Part print with two shaded views. Sizes in mm from the minimum x, y, z corner. Give positions to 0.01 mm unless a question says otherwise; leave off trailing zeros. Loops run counter-clockwise (first coordinate to the right, second up) from the corner with the lowest first, then second, coordinate; pieces in that order, holes last. Notation, with made-up numbers: M -16.5,21.5 L 19.5,21.5 A11 ccw 19.5,39.5 Z; hole C 37,-36.5 d7. An arc over 180 degrees is marked long. Answer in a Markdown table with one row per item.
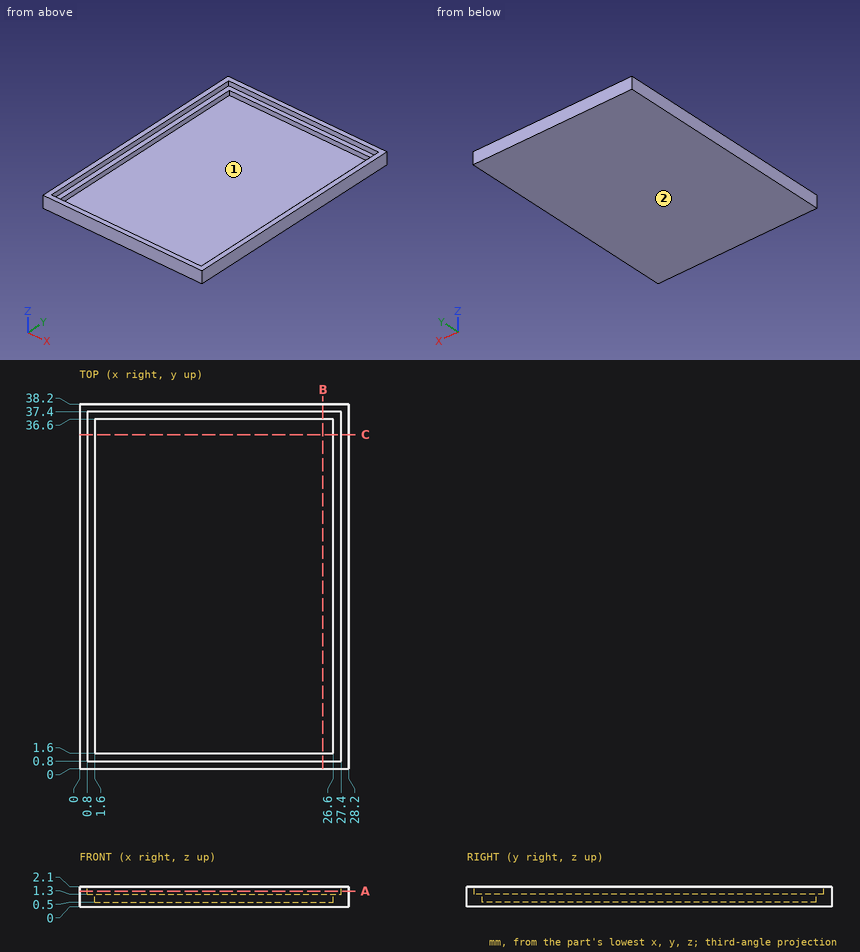
Q1. Saw through at A-A (z = 1.65). Give the cut face in (x, y), and give its area (3 significant figures).
Reported:
| item | result |
|---|---|
| outline | M 0,0 L 28.2,0 L 28.2,38.2 L 0,38.2 Z; hole M 0.8,0.8 L 27.4,0.8 L 27.4,37.4 L 0.8,37.4 Z |
| area | 104 mm² |
Q2. Saw through at B-B (x = 25.5). Give the cut face in (y, z).
Reported:
| item | result |
|---|---|
| outline | M 0,0 L 38.2,0 L 38.2,2.1 L 37.4,2.1 L 37.4,1.3 L 36.6,1.3 L 36.6,0.5 L 1.6,0.5 L 1.6,1.3 L 0.8,1.3 L 0.8,2.1 L 0,2.1 Z |
Q3. Drop flat-ended pins along their axis: pin 1 (1 mm diameter, centred on x = 12.5, z = 0.5, fed in from -Y); pin 2 (3 mm diameter, centred on x = 14.5, y = 24.5, fed in from +Z). Give the stop position or say it passes through.
Reported:
| item | result |
|---|---|
| pin 1 | y = 0 |
| pin 2 | z = 0.5 |
Q4. Probe probe 1 along X at (y, z) = (17.5, 1.4); probe 2 along Y at (x, z) = (23.75, 0.8); probe 3 along Y at (x, z) = (12.25, 1.5). List the from-to ranges inside material, lowest first.
Reported:
| item | result |
|---|---|
| probe 1 | 0 to 0.8, 27.4 to 28.2 |
| probe 2 | 0 to 1.6, 36.6 to 38.2 |
| probe 3 | 0 to 0.8, 37.4 to 38.2 |
Q5. Saw through at C-C (y = 35). Give the cut face in (x, z).
Reported:
| item | result |
|---|---|
| outline | M 0,0 L 28.2,0 L 28.2,2.1 L 27.4,2.1 L 27.4,1.3 L 26.6,1.3 L 26.6,0.5 L 1.6,0.5 L 1.6,1.3 L 0.8,1.3 L 0.8,2.1 L 0,2.1 Z |
Q6. Mould opens along X. For the marked faces 1 and 2 say: released by +X, released by -X, zero draft, split by the parting line, or undercut.
Reported:
| item | result |
|---|---|
| face 1 | undercut |
| face 2 | zero draft |
